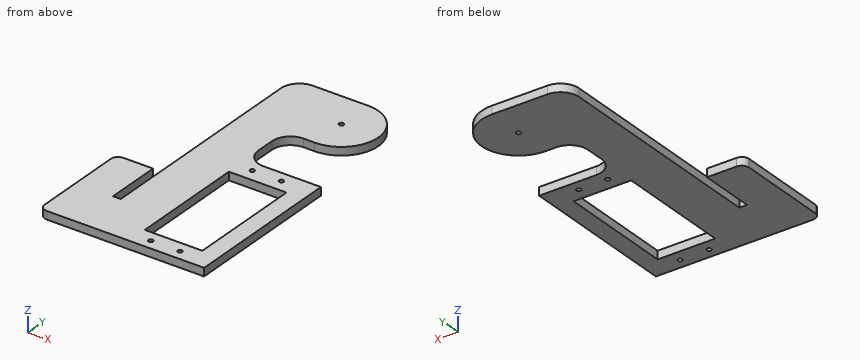
```python
from build123d import *

# Parameters (mm, degrees)
SKETCH1_R           = 0.79375
SKETCH1_W           = 19.812
SKETCH1_H           = 40
BOSS_EXTRUDE1_DEPTH = 2.794
FILLET1_R           = 6.35
FILLET2_R           = 6.35
FILLET5_R           = 2.54


with BuildPart() as part:
    # Sketch1 → Boss-Extrude1 (new body)
    with BuildSketch(Plane.XY):
        with BuildLine():
            Line((-5.842, 4.734159763), (50.8, 4.734159763))
            Line((50.8, 4.734159763), (50.8, 36.343152622))
            Line((50.8, 36.343152622), (50.8, 60.284785263))
            Line((50.8, 60.284785263), (24.765, 60.284785263))
            Line((24.765, 60.284785263), (24.765, 79.327185263))
            Line((24.765, 79.327185263), (34.925, 79.327185263))
            ThreePointArc((34.925, 79.327185263), (47.625, 92.027185263), (34.925, 104.727185263))
            Line((34.925, 104.727185263), (9.525, 104.727185263))
            Line((9.525, 104.727185263), (9.525, 38.1))
            Line((9.525, 38.1), (9.525, 22.177185263))
            Line((9.525, 22.177185263), (6.858, 22.177185263))
            Line((6.858, 22.177185263), (6.858, 41.227185263))
            Line((6.858, 41.227185263), (-5.842, 41.227185263))
            Line((-5.842, 41.227185263), (-5.842, 4.734159763))
        make_face()
        with Locations((34.925, 92.027185263)):
            Circle(SKETCH1_R, mode=Mode.SUBTRACT)
        with Locations((29.9212, 8.283385263)):
            Circle(SKETCH1_R, mode=Mode.SUBTRACT)
        with Locations((39.9288, 8.283385263)):
            Circle(SKETCH1_R, mode=Mode.SUBTRACT)
        with Locations((29.9212, 56.517985263)):
            Circle(SKETCH1_R, mode=Mode.SUBTRACT)
        with Locations((39.9288, 56.517985263)):
            Circle(SKETCH1_R, mode=Mode.SUBTRACT)
        with Locations((34.925, 32.177185263)):
            Rectangle(SKETCH1_W, SKETCH1_H, mode=Mode.SUBTRACT)
    extrude(amount=BOSS_EXTRUDE1_DEPTH)

    # Fillet1
    fillet1_edges = [part.edges().sort_by_distance(p)[0] for p in [
        (24.765, 79.327185263, 1.397),
        (24.765, 60.284785263, 1.397),
    ]]
    fillet(fillet1_edges, radius=FILLET1_R)

    # Fillet2
    fillet2_edges = [part.edges().sort_by_distance(p)[0] for p in [
        (9.525, 104.727185263, 1.397),
    ]]
    fillet(fillet2_edges, radius=FILLET2_R)

    # Fillet5
    fillet5_edges = [part.edges().sort_by_distance(p)[0] for p in [
        (-5.842, 4.734159763, 1.397),
        (-5.842, 41.227185263, 1.397),
    ]]
    fillet(fillet5_edges, radius=FILLET5_R)


solid = part.part
```
Geometry: final body of the model. Coordinates: model frame, mm. Coordinates: 2 decimals unless noted, no trailing zeros. Order: outer loops, then holes, each group sorted by start corner. A loop starts at its lowest first (then second) coordinate and runs counter-clockwise, first axis right, second up. Notation, with made-up numbers: (-36, 42) - (-10, 42) arc R25 ccw to (-10, 58) - close; hole circle Ø11 at (80.25, 1). An arc over 180 degrees is marked (long way). Write each question's results on one line, items separated by ' | '.
1) Section D-D, the plane z = 1.9. State how many separate pieces and enclosed holes the cut face has, plus the area to 3 significant figures.
Results list:
separate pieces: 1 | enclosed holes: 6 | area: 3,200 mm^2
2) Pin query (flat end, axial travel): pin 1 (0.8 mm diameter, centred on x = 2, z = 2, fed in from +Y); pin 2 (1.3 mm diameter, centred on x = 8.5, z = 1, fed in from +Y). Return the tip coordinate at first contact, or that it passes through.
Results list:
pin 1: y = 41.23 | pin 2: y = 22.18
3) Line query: line 1 (X direction, y = 25.5, z = 0.3) (3 decimals); line 2 (Y direction, x = 35, z = 2.7); line 3 (X direction, y = 41.5, z = 0.6) (3 decimals). Output: solid intervals per line, ascending. Write a range as from..to.
Results list:
line 1: -5.842..6.858, 9.525..25.019, 44.831..50.8 | line 2: 4.73..12.18, 52.18..60.28, 79.33..91.24, 92.82..104.73 | line 3: 9.525..25.019, 44.831..50.8
4) Section B-B, the plane y = 27. Return loops of the section in (x, z) (3 decimals).
Results list:
outline: (-5.842, 0) - (6.858, 0) - (6.858, 2.794) - (-5.842, 2.794) - close; (9.525, 0) - (25.019, 0) - (25.019, 2.794) - (9.525, 2.794) - close; (44.831, 0) - (50.8, 0) - (50.8, 2.794) - (44.831, 2.794) - close
5) Section C-C, the plane x = 27.5. Return loops of the section in (y, z), plus the area to 3 significant figures.
Results list:
outline: (4.73, 0) - (12.18, 0) - (12.18, 2.79) - (4.73, 2.79) - close; (52.18, 0) - (61.41, 0) - (61.41, 2.79) - (52.18, 2.79) - close; (78.2, 0) - (104.73, 0) - (104.73, 2.79) - (78.2, 2.79) - close | area: 121 mm^2
6) Section A-A, the plane y = 46.5. Return loops of the section in (x, z) (3 decimals).
Results list:
outline: (9.525, 0) - (25.019, 0) - (25.019, 2.794) - (9.525, 2.794) - close; (44.831, 0) - (50.8, 0) - (50.8, 2.794) - (44.831, 2.794) - close
